Source: CAD feature listing. Evaluate the final solid. Frame: model axes, mm. A direction names the side the tool comes from. Give positions to 0.01 mm unless a question says otherwise; leave off trailing zeros. Loops run counter-clockwise (first coordinate to the right, second up) from the corner with the lowest first, then second, coordinate; pieces in that order, holes last. Notation, with made-up numbers: M -33.5,3.25 L 18.5,3.25 A15 cw 18.5,24.25 Z; hole C -17.5,19 d7. An arc over 180 degrees is marked long. Put each result on its own line as item: value. Start each with the question number.
Autodesk Inventor part; units mm, degrees
sketch "Эскиз1" plane through (0, 0, 0) normal (0, 1, 0) x (-1, 0, 0)
  line L0 (35, 120) -> (-35, 120)
  line L1 (-35, 120) -> (-35, -120)
  line L2 (-35, -120) -> (35, -120)
  line L3 (35, -120) -> (35, 120)
  line L4 (35, 120) -> (-35, -120) construction
  line L5 (-35, 120) -> (35, -120) construction
  point P0 (0, 0)
  dimension "d0" = 70
  dimension "d1" = 240
extrude "Выдавливание1" add sketch "Эскиз1" along normal mid plane 10
shell "Оболочка1" thickness 3 outward yes removed faces 1 at (-11.6667, -5, -40)
sketch "Эскиз2" plane through (0, 8, 0) normal (0, 1, 0) x (1, 0, 0)
  line L0 (0, 85) -> (0, -85) construction
  line L1 (-27.5, 85) -> (-27.5, -85)
  line L2 (27.5, -85) -> (27.5, 85)
  arc A0 (27.5, 85) -> (-27.5, 85) centre (0, 85) ccw
  arc A1 (-27.5, -85) -> (27.5, -85) centre (0, -85) ccw
  point P0 (0, 0)
  point P1 (0, -112.5)
  point P2 (0, 112.5)
  dimension "d5" = 225
  dimension "d6" = 55
extrude "Выдавливание2" cut sketch "Эскиз2" against normal up to next
properties part number "Крышка_крепления_динамика"
1. Section B-B, the plane x = 0. Output: boundary loops of the cut face in (y, z), plus the area to 3 significant figures.
2. Ray query, line 1 (X direction, y = -2, z = 102.5); line 2 (Z direction, x = 34.5, y = -4.5); line 3 (X direction, y = 5.75, z = -30). Return the intervals inside material, ascending.
3. Contact query for a flat-ended pin moving along its axis: pin 1 (4 mm diameter, centred on x = -24, z = 29, fed in from -Y). Output: stop coordinate, or through.
4. Section A-A, the plane y = 1. Output: boundary loops of the cut face in (x, z), plus the area to 3 significant figures.
5. Set-up query: faces 4 (the face through (0.605, 6.521, -112.493)), 5 (the face through (-36, -5, 1)), 6 (the face through (35, 0, 2)). Return all of +Z, -Z, +X, -X, +Y, -Y with unobstructed straight access to the full face (end or side cutting, diameter ignored); none if empty.
6. Pull-direction query (Z, two-part tool) for faces 1 (the face through (38, 1, 2)), 2 (the face through (0, 0, -120)), 3 (the face through (1, 1, -123)); classes: released by +Z, released by -Z, zero draft, split by the parting line, or undercut.
7. Section C-C, the plane z = 51. Output: boundary loops of the cut face in (x, y).
Results found:
1. outline: M -5,-123 L 8,-123 L 8,-112.5 L 5,-112.5 L 5,-120 L -5,-120 Z; M -5,120 L 5,120 L 5,112.5 L 8,112.5 L 8,123 L -5,123 Z
1. area: 123 mm²
2. line 1: -38 to -35, 35 to 38
2. line 2: -123 to -120, 120 to 123
2. line 3: -38 to -27.5, 27.5 to 38
3. pin 1: through
4. outline: M -38,-123 L 38,-123 L 38,123 L -38,123 Z; hole M -35,-120 L 35,-120 L 35,120 L -35,120 Z
4. area: 1,900 mm²
5. face 4: +Y, -Y
5. face 5: +Z, -Z, +X, -X, -Y
5. face 6: -Y
6. face 1: zero draft
6. face 2: undercut
6. face 3: released by -Z
7. outline: M -38,-5 L -35,-5 L -35,5 L -27.5,5 L -27.5,8 L -38,8 Z; M 27.5,5 L 35,5 L 35,-5 L 38,-5 L 38,8 L 27.5,8 Z
